Source: CAD feature listing. Evaluate the final solid. Frame: model axes, mm. Face numbers are marked on the shaded views. A direction names the side the tool comes from. Coordinates: 2 decimals unless noted, no trailing zeros. Order: outer loops, then holes, each group sorted by start corner. A loop starts at its lowest first (then second) coordinate and runs counter-clockwise, first axis right, second up. Notation, with made-up numbers: (50, 33) - (60, 33) arc R18 cw to (60, 46) - close; hole circle Ø1 at (-12.5, 72). An arc over 180 degrees is marked (long way). One line per question, with ' | ' between items. Start each with the question number.
(1) Draft query along X for the marked faces 1, 2 and 3. Return one class per face: +X half, -X half, draft (parallel to the pull), parting line (faces both ways), or undercut.
(2) Access query for the marked faces 4, 5, 6 and 7. Directions: +Z, -Z, +X, -X, +Y, -Y. A direction counts if a zero-diameter tool reaches every point of the face in a straight line with its end or side. Return the directions, or none.
(3) Section C-C (z = 16.5). Return the cut outline in (x, y).
(4) Section B-B (x = 101.6). Return the cut outline in (y, z), then the cut area to 3 significant figures.
(5) Section A-A (y = -25). Return the cut outline in (x, z), then the cut area to 3 significant figures.
(6) Contact query for flat-ended pins moving along their axis: P1, Ø5.5, axis at x = 40, y = -8.5, coming from the +Z side; P2, Ø1.5, axis at x = 39, z = 7, coming from the +Y side; P3, Ø6, axis at x = 150.5, z = 13, coming from the +Y side. Output: stop coordinate, or through.
(7) Line query: line 1 along X through (y, z) = (-11, 25); line 2 along Z through (x, y) = (208, -8.5); line 3 along Y through (x, z) = (233, 30). Output: solid intervals per line, ascending.
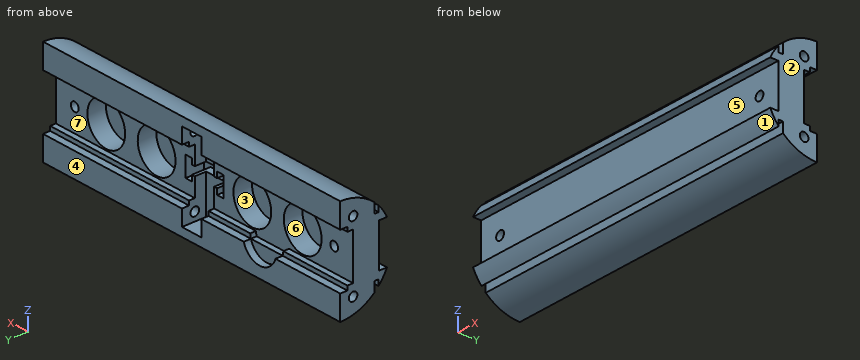
from build123d import *

# Parameters (mm, degrees)
SLED_DEPTH                       = 299.72
SKETCH12_R                       = 19.05
SPRING_INSERTS_DEPTH             = 27.94
SKETCH4_R                        = 3.81
THREADED_ROD_SLOTS_DEPTH         = 304.8
SKETCH13_W                       = 19.558
SKETCH13_H                       = 76.2
SPRING_PLATE_SLOT_DEPTH          = 21.59
MOD_TO_FIT_IN_COUPLER_DEPTH      = 320.04
MOD_TO_FIT_IN_COUPLER_DEPTH_BACK = 77.47
SKETCH17_R                       = 3.937
CAN_CORD_HOLES_DEPTH             = 62.992
INSERTION_GUIDE_RAILS_DEPTH      = 314.452
LOCKING_PIN_DEPTH                = 27.94
SKETCH20_R                       = 16.764
CUT_EXTRUDE1_DEPTH               = 6.35
CUT_EXTRUDE2_DEPTH               = 11.43


with BuildPart() as part:
    # Sketch3 → Sled (new body)
    with BuildSketch(Plane(origin=(0, 0, 0), x_dir=(0, 0, -1), z_dir=(1, 0, 0))):
        with BuildLine():
            Line((-49.53, 0), (-24.13, 0))
            Line((-24.13, 0), (-24.13, -6.35))
            Line((-24.13, -6.35), (-20.32, -6.35))
            Line((-20.32, -6.35), (-20.32, -11.43))
            Line((-20.32, -11.43), (20.32, -11.43))
            Line((20.32, -11.43), (20.32, -6.35))
            Line((20.32, -6.35), (24.13, -6.35))
            Line((24.13, -6.35), (24.13, 0))
            Line((24.13, 0), (49.53, 0))
            ThreePointArc((49.53, 0), (41.211451079, -27.474300719), (19.05, -45.72))
            Line((19.05, -45.72), (19.05, -34.29))
            Line((19.05, -34.29), (-19.05, -34.29))
            Line((-19.05, -34.29), (-19.05, -45.72))
            ThreePointArc((-19.05, -45.72), (-41.211451079, -27.474300719), (-49.53, 0))
        make_face()
    extrude(amount=SLED_DEPTH)

    # Sketch12 → Spring Inserts (cut)
    with BuildSketch(Plane(origin=(0, 0, 0), x_dir=(1, 0, 0), z_dir=(0, 1, 0))):
        with Locations(Location((50.8, 0, 0), (0, 0, 270))):
            Circle(SKETCH12_R)
        with Locations(Location((248.92, 0, 0), (0, 0, 90))):
            Circle(SKETCH12_R)
        with Locations(Location((101.6, 0, 0), (0, 0, 270))):
            Circle(SKETCH12_R)
        with Locations(Location((198.12, 0, 0), (0, 0, 90))):
            Circle(SKETCH12_R)
    extrude(amount=-SPRING_INSERTS_DEPTH, mode=Mode.SUBTRACT)

    # Sketch4 → Threaded Rod Slots (cut)
    with BuildSketch(Plane(origin=(0, 0, 0), x_dir=(0, 0, -1), z_dir=(1, 0, 0))):
        with Locations(Location((-30.48, -11.43, 0), (0, 0, 180))):
            Circle(SKETCH4_R)
        with Locations(Location((30.48, -11.43, 0), (0, 0, 180))):
            Circle(SKETCH4_R)
    extrude(amount=THREADED_ROD_SLOTS_DEPTH, mode=Mode.SUBTRACT)

    # Sketch13 → Spring Plate Slot (cut)
    with BuildSketch(Plane(origin=(0, 0, 0), x_dir=(1, 0, 0), z_dir=(0, 1, 0))):
        with Locations((149.86, 0)):
            Rectangle(SKETCH13_W, SKETCH13_H)
    extrude(amount=-SPRING_PLATE_SLOT_DEPTH, mode=Mode.SUBTRACT)

    # Sketch16 → Mod to fit in coupler (cut, two sides: drawn at the far end of the back side and taken through both)
    with BuildSketch(Plane(origin=(0, 0, 0), x_dir=(0, 0, -1), z_dir=(1, 0, 0)).offset(-MOD_TO_FIT_IN_COUPLER_DEPTH_BACK)):
        with BuildLine():
            Line((-45.397424247, 5.421463987), (-55.982128016, 1.685686186))
            Line((-55.982128016, 1.685686186), (-46.435140302, -53.451626912))
            Line((-46.435140302, -53.451626912), (-2.643522748, -59.401198965))
            Line((-2.643522748, -59.401198965), (46.059950804, -46.118433451))
            Line((46.059950804, -46.118433451), (57.336465277, 3.138488664))
            Line((57.336465277, 3.138488664), (45.312886192, 6.087753686))
            ThreePointArc((45.312886192, 6.087753686), (0.335815666, -45.718766692), (-45.397424247, 5.421463987))
        make_face()
    extrude(amount=MOD_TO_FIT_IN_COUPLER_DEPTH + MOD_TO_FIT_IN_COUPLER_DEPTH_BACK, mode=Mode.SUBTRACT)

    # Sketch17 → Can Cord Holes (cut)
    with BuildSketch(Plane(origin=(0, 0, 0), x_dir=(1, 0, 0), z_dir=(0, 1, 0))):
        with Locations(Location((280.67, 0, 0), (0, 0, 270))):
            Circle(SKETCH17_R)
        with Locations(Location((19.05, 0, 0), (0, 0, 270))):
            Circle(SKETCH17_R)
    extrude(amount=-CAN_CORD_HOLES_DEPTH, mode=Mode.SUBTRACT)

    # Sketch18 → Insertion Guide Rails (cut)
    with BuildSketch(Plane(origin=(0, 0, 0), x_dir=(0, 0, -1), z_dir=(1, 0, 0))):
        Polygon((-34.29, -30.240937485), (-25.4, -30.240937485), (-25.4, -34.050937485), (-30.50986818, -34.050937485), (-38.766826884, -32.646576067), align=None)
        Polygon((25.4, -34.050937485), (30.50986818, -34.050937485), (38.766826884, -32.646576067), (34.29, -30.240937485), (25.4, -30.240937485), align=None)
    extrude(amount=INSERTION_GUIDE_RAILS_DEPTH, mode=Mode.SUBTRACT)

    # Sketch19 → Locking Pin (cut)
    with BuildSketch(Plane(origin=(0, 0, 0), x_dir=(1, 0, 0), z_dir=(0, 1, 0))):
        Polygon((162.56, 3.81), (137.16, 3.81), (137.16, 8.89), (130.81, 8.89), (130.81, -8.89), (137.16, -8.89), (137.16, -3.81), (162.56, -3.81), (162.56, -8.89), (168.91, -8.89), (168.91, 8.89), (162.56, 8.89), align=None)
    extrude(amount=-LOCKING_PIN_DEPTH, mode=Mode.SUBTRACT)

    # Sketch20 → Cut-Extrude1 (cut)
    with BuildSketch(Plane(origin=(0, 0, 0), x_dir=(1, 0, 0), z_dir=(0, 1, 0))):
        with Locations((81.28, 19.05)):
            Circle(SKETCH20_R)
    extrude(amount=-CUT_EXTRUDE1_DEPTH, mode=Mode.SUBTRACT)

    # Sketch21 → Cut-Extrude2 (cut)
    with BuildSketch(Plane(origin=(0, 0, 0), x_dir=(1, 0, 0), z_dir=(0, 1, 0))):
        with BuildLine():
            Line((97.266479016, 24.096204976), (65.284485664, 24.067491117))
            ThreePointArc((65.284485664, 24.067491117), (81.295050936, 2.286006756), (97.266479016, 24.096204976))
        make_face()
    extrude(amount=-CUT_EXTRUDE2_DEPTH, mode=Mode.SUBTRACT)


solid = part.part
Response values:
1) face 1: draft | face 2: +X half | face 3: undercut
2) face 4: +Z, -Z, +X, -X, +Y | face 5: +X, -X, -Y | face 6: +Y | face 7: +X, -X, +Y
3) outline: (0, -34.29) - (299.72, -34.29) - (299.72, -11.43) - (258.44, -11.43) - (258.44, -27.94) - (239.4, -27.94) - (239.4, -11.43) - (207.64, -11.43) - (207.64, -27.94) - (188.6, -27.94) - (188.6, -11.43) - (159.64, -11.43) - (159.64, -21.59) - (140.08, -21.59) - (140.08, -11.43) - (111.12, -11.43) - (111.12, -27.94) - (92.08, -27.94) - (92.08, -11.43) - (60.32, -11.43) - (60.32, -27.94) - (41.28, -27.94) - (41.28, -11.43) - (0, -11.43) - close
4) outline: (-41.56, -19.05) arc R45.72 ccw to (-34.05, -30.51) - (-34.05, -25.4) - (-30.24, -25.4) - (-30.24, -34.29) arc R45.72 ccw to (0, -45.72) - (0, -24.13) - (-6.35, -24.13) - (-6.35, -20.32) - (-11.43, -20.32) - (-11.43, -19.05) - (-27.94, -19.05) - (-27.94, 19.05) - (-11.43, 19.05) - (-11.43, 20.32) - (-6.35, 20.32) - (-6.35, 24.13) - (0, 24.13) - (0, 45.72) arc R45.72 ccw to (-30.24, 34.29) - (-30.24, 25.4) - (-34.05, 25.4) - (-34.05, 30.51) arc R45.72 ccw to (-41.56, 19.05) - (-34.29, 19.05) - (-34.29, -19.05) - close; hole circle Ø7.62 at (-11.43, -30.48); hole circle Ø7.62 at (-11.43, 30.48) | area: 1,610 mm²
5) outline: (0, -38.28) - (299.72, -38.28) - (299.72, 38.28) - (0, 38.28) - close; hole circle Ø7.87 at (19.05, 0); hole circle Ø38.1 at (50.8, 0); hole circle Ø38.1 at (101.6, 0); hole (130.81, -8.89) - (137.16, -8.89) - (137.16, -3.81) - (162.56, -3.81) - (162.56, -8.89) - (168.91, -8.89) - (168.91, 8.89) - (162.56, 8.89) - (162.56, 3.81) - (137.16, 3.81) - (137.16, 8.89) - (130.81, 8.89) - close; hole circle Ø38.1 at (198.12, 0); hole circle Ø38.1 at (248.92, 0); hole circle Ø7.87 at (280.67, 0) | area: 17,900 mm²
6) P1: stops at z = 45.36 | P2: stops at y = -27.94 | P3: stops at y = -21.59
7) line 1: x = 0 to 140.08, 159.64 to 299.72 | line 2: z = -44.92 to -32.92, -28.04 to -20.32, 20.32 to 28.04, 32.92 to 44.92 | line 3: y = -34.5 to -34.05, -30.24 to -15.21, -7.65 to 0
